from build123d import *

# Parameters (mm, degrees)
SKETCH1_R           = 2.5
BOSS_EXTRUDE1_DEPTH = 2
BOSS_EXTRUDE2_DEPTH = 2
BOSS_EXTRUDE3_DEPTH = 16
BOSS_EXTRUDE4_START = 2
SKETCH5_R           = 2.5
BOSS_EXTRUDE4_DEPTH = 2


with BuildPart() as part:
    # Sketch1 → Boss-Extrude1 (new body)
    with BuildSketch(Plane(origin=(0, 0, 0), x_dir=(1, 0, 0), z_dir=(0, 1, 0))):
        with BuildLine():
            Line((0, 5), (20, 5))
            ThreePointArc((20, 5), (25, 0), (20, -5))
            Line((20, -5), (0, -5))
            ThreePointArc((0, -5), (-5, 0), (0, 5))
        make_face()
        with Locations(Location((0, 0, 0), (0, 0, 270))):
            Circle(SKETCH1_R, mode=Mode.SUBTRACT)
        with Locations(Location((20, 0, 0), (0, 0, 270))):
            Circle(SKETCH1_R, mode=Mode.SUBTRACT)
    extrude(amount=BOSS_EXTRUDE1_DEPTH)

    # Sketch3 → Boss-Extrude2 (add)
    with BuildSketch(Plane(origin=(0, 2, 0), x_dir=(1, 0, 0), z_dir=(0, 1, 0))):
        Polygon((20, 5), (48.392339972, -4.000005434), (51.150724408, 4.055463463), (79.532873786, -5.663260562), (77.913086448, -10.393618791), (33.419519193, -10.393618791), (20, -5), (24.317409575, 2.521898999), align=None)
    extrude(amount=-BOSS_EXTRUDE2_DEPTH)

    # Sketch4 → Boss-Extrude3 (add)
    with BuildSketch(Plane.XZ):
        Polygon((51.150724408, -4.055463463), (79.532873786, 5.663260562), (78.884958851, 7.555403854), (50.502809473, -2.163320171), align=None)
    extrude(amount=BOSS_EXTRUDE3_DEPTH)

    # Sketch5 → Boss-Extrude4 (add)
    with BuildSketch(Plane.XZ.offset(16).offset(BOSS_EXTRUDE4_START)):
        with BuildLine():
            Line((48.392339972, 4.000005434), (51.150724408, -4.055463463))
            Line((51.150724408, -4.055463463), (79.532873786, 5.663260562))
            Line((79.532873786, 5.663260562), (77.913086448, 10.393618791))
            Line((77.913086448, 10.393618791), (33.419519193, 10.393618791))
            Line((33.419519193, 10.393618791), (20, 5))
            Line((20, 5), (0, 5))
            ThreePointArc((0, 5), (-5, 0), (0, -5))
            Line((0, -5), (20, -5))
            ThreePointArc((20, -5), (20.764409298, -4.941222361), (21.510846527, -4.76627137))
            Line((21.510846527, -4.76627137), (21.589436532, -4.740642521))
            Line((21.589436532, -4.740642521), (48.392339972, 4.000005434))
        make_face()
        with Locations(Location((0, 0, 0), (0, 0, 90))):
            Circle(SKETCH5_R, mode=Mode.SUBTRACT)
        with Locations(Location((20, 0, 0), (0, 0, 270))):
            Circle(SKETCH5_R, mode=Mode.SUBTRACT)
    extrude(amount=-BOSS_EXTRUDE4_DEPTH)


solid = part.part
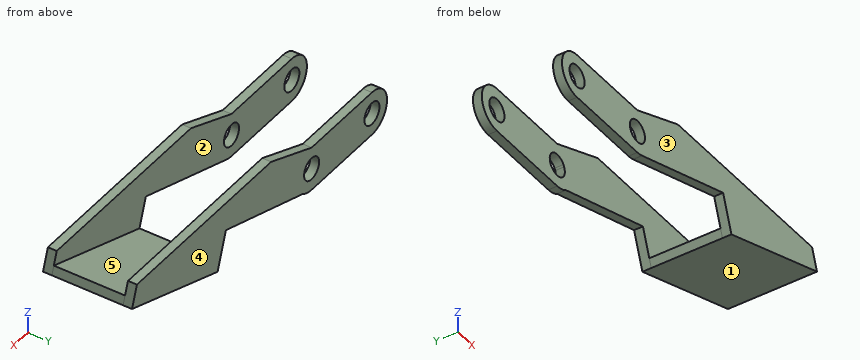
The model under review builds one solid part; all positions refer to its coordinate system, in mm. Face numbers are marked on the shaded views. A direction names the side the tool comes from. Coordinates: 2 decimals unless noted, no trailing zeros. Loops run counter-clockwise (first coordinate to the right, second up) from the corner with the lowest first, then second, coordinate; pieces in that order, holes last.
(1) Tool access review of the marked faces 1 and 2: name each direction out of +Z, -Z, +X, -X, +Y, -Y from which nothing blocks a thin tool from reaching the whole face with its end or side.
Determined:
face 1: -Z, +X, +Y, -Y
face 2: +Z, -X
(2) Consider section A-A, the plane x = 1.5. Give the boundary of the cut face in (y, z).
Determined:
outline: (-18, -5) - (-16, -5) - (-16, -2) - (-18, -2) - close; (-18, 2) - (-16, 2) - (-16, 5) - (-18, 5) - close; (0, -5) - (2, -5) - (2, -2) - (0, -2) - close; (0, 2) - (2, 2) - (2, 5) - (0, 5) - close
(3) Draft analysis for pull direction Y (two halves, no side actions). For the marked faces 3, 4 and 5, state which applies: +Y half, -Y half, draft (parallel to the pull), parting line (faces both ways), or undercut.
Determined:
face 3: -Y half
face 4: +Y half
face 5: undercut
(4) Consider section B-B, the plane z = 0. Give the number of separate pieces and of enclosed holes in the cut face, plus the area to 3 significant figures.
Determined:
separate pieces: 7
enclosed holes: 0
area: 276 mm2
(5) Consider section C-C, the plane x = 40.5. Give the boundary of the cut face in (y, z), plus the area to 3 significant figures.
Determined:
outline: (-18, 1.43) - (-16, 1.43) - (-16, 10.39) - (-18, 10.39) - close; (0, 1.5) - (2, 1.5) - (2, 10.39) - (0, 10.39) - close
area: 35.7 mm2
(6) Wall thickness on L1, parallel to Y at x = 14, z = 1.5; L2, parallel to Z at x = 20, y = 0.5; L3, parallel to Z at x = 69.5, y = -6.75: over which ranges is each line inside the solid? List them lowest first.
Determined:
L1: y = -18 to -16, 0 to 2
L2: z = -5 to -2.5, 2.5 to 5
L3: z = 2.23 to 4.34
(7) Insertion check: P1, Ø12, axis at x = 21, y = -15, coming from the +Z side; P2, Ø0.6, axis at x = 9, y = 0.5, coming from the +Z side; P3, Ø12, axis at x = 34.5, y = -14.5, coming from the -Z side. Each pin has a flat end and moves straight along its axis. Give the tip position at first contact, or say it passes through.
Determined:
P1: stops at z = 7.78
P2: stops at z = 5
P3: stops at z = -2.42
(8) Consider section D-D, the plane x = 74. Give the boundary of the cut face in (y, z).
Determined:
outline: (-18, 3.77) - (2, 3.77) - (2, 10.39) - (0, 10.39) - (0, 5.88) - (-16, 5.88) - (-16, 10.39) - (-18, 10.39) - close
